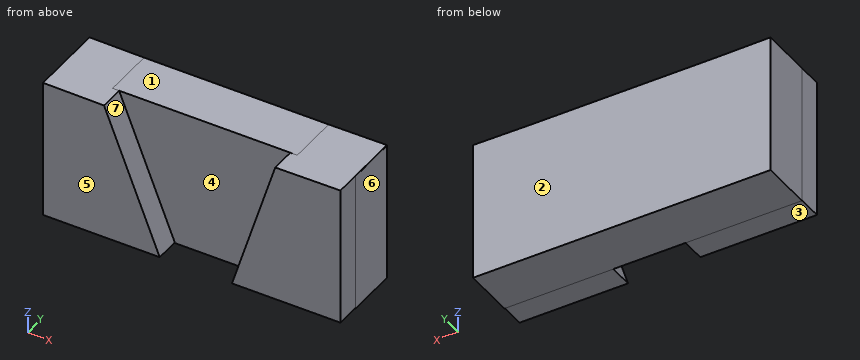
```python
from build123d import *

# Parameters (mm, degrees)
F0_W     = 146.320656
F0_H     = 69.079675
F2_DEPTH = 25.4
F3_DEPTH = 37.592


with BuildPart() as f2:
    # F0 (on Front) → F2 (new body)
    with BuildSketch(Plane.XZ):
        with Locations((0, -3.206231)):
            Rectangle(F0_W, F0_H)
    extrude(amount=F2_DEPTH)

    # F1 (on Front) → F3 (join)
    with BuildSketch(Plane.XZ):
        Polygon((-43.118302, 31.302609), (-73.125824, 31.593941), (-73.125824, -37.452485), (-15.732799, -37.452485), align=None)
        Polygon((73.124416, -37.452485), (73.124416, 31.593941), (41.077554, 31.302609), (19.810088, -37.452485), align=None)
    extrude(amount=F3_DEPTH)


solid = f2.part
```
Source: CAD feature listing. Evaluate the final solid. Frame: model axes, mm. Face numbers are marked on the shaded views. A direction names the side the tool comes from. Give positions to 0.01 mm unless a question says otherwise; leave off trailing zeros. Order: outer loops, then holes, each group sorted by start corner. A loop starts at its lowest first (then second) coordinate and runs counter-clockwise, first axis right, second up.
(1) Section query A-A (y = -33). Return the cut outline in (x, z), plus the area to 3 significant figures.
(2) Section query C-C (x = -39). Return the cut outline in (y, z), plus the area to 3 significant figures.
(3) Material intervals for line 1 along Y through (x, z) = (-15, -8); line 2 along X through (y, z) = (-28, -4.5); line 3 along Z through (x, y) = (35.5, -16), sorted ascending.
(4) Access query for the marked faces 1, 2 and 3. Directions: +Z, -Z, +X, -X, +Y, -Y. A direction counts if a zero-diameter tool reaches every point of the face in a straight line with its end or side. Return the directions, or none.
(5) Contact query for flat-ended pins moving along their axis: P1, Ø12, axis at x = 7.5, z = 3.5, coming from the -Y side; P2, Ø2, axis at x = -45, y = -15.5, coming from the +Z side. Output: stop coordinate, or through.
(6) Pull-direction query (X, two-part tool) for the marked faces 4, 5, 6 and 7; classes: +X half, -X half, draft (parallel to the pull), parting line (faces both ways), or undercut.
(7) Section query D-D (x = 35). Return the cut outline in (y, z).
Outcome:
1. outline: (-73.13, -37.45) - (-15.73, -37.45) - (-43.12, 31.3) - (-73.13, 31.59) - close; (19.81, -37.45) - (73.12, -37.45) - (73.12, 31.59) - (41.08, 31.3) - close
1. area: 5,950 mm2
2. outline: (-37.59, -37.45) - (-25.4, -37.45) - (-25.4, -37.75) - (0, -37.75) - (0, 31.33) - (-25.4, 31.33) - (-25.4, 20.96) - (-37.59, 20.96) - close
2. area: 2,470 mm2
3. line 1: y = -25.4 to 0
3. line 2: x = -73.13 to -28.86, 30 to 73.12
3. line 3: z = -37.75 to 31.33
4. face 1: +Z, +Y, -Y
4. face 2: +Z, -Z, +X, -X, +Y
4. face 3: -Z, +X, -X, -Y
5. P1: stops at y = -25.4
5. P2: stops at z = 31.33
6. face 4: undercut
6. face 5: draft
6. face 6: +X half
6. face 7: undercut
7. outline: (-37.59, -37.45) - (-25.4, -37.45) - (-25.4, -37.75) - (0, -37.75) - (0, 31.33) - (-25.4, 31.33) - (-25.4, 11.65) - (-37.59, 11.65) - close
